```python
from build123d import *

# Parameters (mm, degrees)
F1_DEPTH = 25.4
F2_R     = 6.35
F3_DEPTH = 25.4
F4_R     = 6.35
F5_DEPTH = 49.276
F6_R     = 6.35
F7_DEPTH = 25.4


with BuildPart() as f1:
    # F0 (on Front) → F1 (new body)
    with BuildSketch(Plane.XZ):
        Polygon((0, 12.7), (0, 0), (101.6, 0), (101.6, 12.7), (69.85, 12.7), (69.85, 50.8), (31.75, 50.8), (31.75, 12.7), align=None)
    extrude(amount=-F1_DEPTH)

    # F2 (on face) → F3 (cut)
    with BuildSketch(Plane.XY.offset(12.7)):
        with Locations((82.55, 12.7)):
            Circle(F2_R)
        with BuildLine():
            ThreePointArc((82.55, 25.4), (95.25, 12.7), (82.55, 0))
            Line((82.55, 0), (101.6, 0))
            Line((101.6, 0), (101.6, 25.4))
            Line((101.6, 25.4), (82.55, 25.4))
        make_face()
    extrude(amount=-F3_DEPTH, mode=Mode.SUBTRACT)

    # F4 (on face) → F5 (cut)
    with BuildSketch(Plane.YZ.offset(69.85)):
        with Locations((12.7, 38.1)):
            Circle(F4_R)
        with BuildLine():
            ThreePointArc((12.7, 50.8), (21.680256, 47.080256), (25.4, 38.1))
            Line((25.4, 38.1), (25.4, 50.8))
            Line((25.4, 50.8), (12.7, 50.8))
        make_face()
        with BuildLine():
            ThreePointArc((0, 38.1), (3.719744, 47.080256), (12.7, 50.8))
            Line((12.7, 50.8), (0, 50.8))
            Line((0, 50.8), (0, 38.1))
        make_face()
    extrude(amount=-F5_DEPTH, mode=Mode.SUBTRACT)

    # F6 (on face) → F7 (cut)
    with BuildSketch(Plane.XY.offset(12.7)):
        with BuildLine():
            ThreePointArc((19.05, 0), (6.35, 12.7), (19.05, 25.4))
            Line((19.05, 25.4), (0, 25.4))
            Line((0, 25.4), (0, 0))
            Line((0, 0), (19.05, 0))
        make_face()
        with Locations((19.05, 12.7)):
            Circle(F6_R)
    extrude(amount=-F7_DEPTH, mode=Mode.SUBTRACT)


solid = f1.part
```
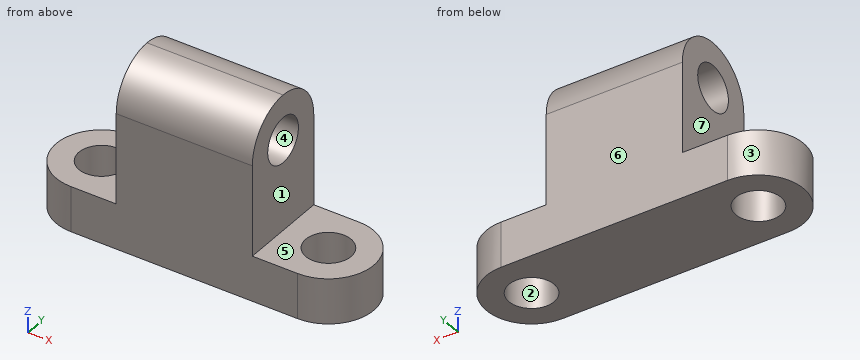
For this review, take the finished solid that the model builds, in its own axes (mm). Face numbers are marked on the shaded views. A direction names the side the tool comes from. Give positions to 0.01 mm unless a question says otherwise; leave off trailing zeros. Write each loop counter-clockwise with the first axis right and the second up, starting at its lowest first coordinate (ties: lowest second). Pieces come first, ordered by that corner, then holes.
Item 1: Wall thickness on probe 1 along Y at (x, z) = (82.55, 6.75); probe 2 along Z at (x, y) = (42.5, 12.7); probe 3 along X at (y, z) = (8.5, 9.5): over which ranges is each line inside the solid? List them lowest first.
Item 2: The part is to be moulded in two halves that separate along Y. For the marked faces 1, 2, 3 and 4, say which applies: +Y half, -Y half, draft (parallel to the pull), parting line (faces both ways), or undercut.
Item 3: Take a section at B-B (x = 22). Give the boundary of the cut face in (y, z), and give its area (3 significant figures).
Item 4: Machinability: for the marked faces 5, 6 and 7, which of the approach directions +Z, -Z, +X, -X, +Y, -Y give a long, thin tool a straight path to every point of the face, cutting with its end or side? Answer none if there is none.
Item 5: Take a section at C-C (z = 34.5). Give the boundary of the cut face in (x, y).
Item 6: Take a section at A-A (x = 66.5). Give the boundary of the cut face in (y, z), and give its area (3 significant figures).
Item 7: Take a section at D-D (y = 15.25). Give the boundary of the cut face in (x, z).
Item 8: Insertion check: P1, Ø2, axis at x = 37.5, y = 20, coming from the -Z side; P2, Ø7.5, axis at x = 87, y = 14.5, coming from the +Z side; P3, Ø12.5, axis at y = 9, z = 28.5, coming from the -X side; P4, Ø3, axis at x = 57.5, z = 40, coming from the +Y side. Each pin has a flat end and moves straight along its axis. Give the tip position at first contact, or say it passes through.
Established:
1. probe 1: y = 0 to 6.35, 19.05 to 25.4
1. probe 2: z = 0 to 31.75, 44.45 to 50.8
1. probe 3: x = 7.06 to 14.29, 23.81 to 77.79, 87.31 to 94.54
2. face 1: draft
2. face 2: undercut
2. face 3: parting line
2. face 4: undercut
3. outline: (0, 0) - (7.08, 0) - (7.08, 12.7) - (0, 12.7) - close; (18.32, 0) - (25.4, 0) - (25.4, 12.7) - (18.32, 12.7) - close
3. area: 180 mm2
4. face 5: +Z, +X, +Y, -Y
4. face 6: +Z, -Z, +X, -X, +Y
4. face 7: +Z, -X, +Y, -Y
5. outline: (31.75, 0) - (69.85, 0) - (69.85, 7.47) - (31.75, 7.47) - close; (31.75, 17.93) - (69.85, 17.93) - (69.85, 25.4) - (31.75, 25.4) - close
6. outline: (0, 0) - (25.4, 0) - (25.4, 38.1) arc R12.7 ccw to (0, 38.1) - close; hole circle Ø12.7 at (12.7, 38.1)
6. area: 1,090 mm2
7. outline: (6.61, 0) - (13.23, 0) - (13.23, 12.7) - (6.61, 12.7) - close; (24.87, 0) - (76.73, 0) - (76.73, 12.7) - (69.85, 12.7) - (69.85, 32.28) - (31.75, 32.28) - (31.75, 12.7) - (24.87, 12.7) - close; (31.75, 43.92) - (69.85, 43.92) - (69.85, 50.54) - (31.75, 50.54) - close; (88.37, 0) - (94.99, 0) - (94.99, 12.7) - (88.37, 12.7) - close
8. P1: stops at z = 0
8. P2: stops at z = 12.7
8. P3: stops at x = 31.75
8. P4: stops at y = 25.39
